Geometry check sheet. Reference: the model listing, model coordinates, mm. A direction names the side the tool comes from. Round coordinates to 2 decimals unless told otherwise and drop trailing zeros. Loops run counter-clockwise (first coordinate to the right, second up) from the corner with the lowest first, then second, coordinate; pieces in that order, holes last. Notation, with made-up numbers: (75, -4) - (119, -4) arc R30 ccw to (119, 22) - close; hole circle Ø5 at (21, 51). An arc over 180 degrees is marked (long way). Write item = value, one per line.
```python
from build123d import *

# Parameters (mm, degrees)
SKETCH1_R           = 49.53
SKETCH1_R_2         = 2.15265
SKETCH1_R_3         = 17.4625
SKETCH1_R_4         = 3.175
BOSS_EXTRUDE1_DEPTH = 3.175
CUT_EXTRUDE1_DEPTH  = 71.117918002


with BuildPart() as part:
    # Sketch1 → Boss-Extrude1 (new body)
    with BuildSketch(Plane(origin=(0, 0, 0), x_dir=(0, 0, -1), z_dir=(1, 0, 0))):
        Circle(SKETCH1_R)
        with Locations((0, 45.085)):
            Circle(SKETCH1_R_2, mode=Mode.SUBTRACT)
        with Locations((31.87990923, 31.87990923)):
            Circle(SKETCH1_R_2, mode=Mode.SUBTRACT)
        with Locations((45.085, 0)):
            Circle(SKETCH1_R_2, mode=Mode.SUBTRACT)
        with Locations((31.87990923, -31.87990923)):
            Circle(SKETCH1_R_2, mode=Mode.SUBTRACT)
        with Locations((0, -45.085)):
            Circle(SKETCH1_R_2, mode=Mode.SUBTRACT)
        with Locations((-31.87990923, -31.87990923)):
            Circle(SKETCH1_R_2, mode=Mode.SUBTRACT)
        with Locations((-45.085, 0)):
            Circle(SKETCH1_R_2, mode=Mode.SUBTRACT)
        with Locations((-31.87990923, 31.87990923)):
            Circle(SKETCH1_R_2, mode=Mode.SUBTRACT)
        Circle(SKETCH1_R_3, mode=Mode.SUBTRACT)
        with Locations((9.720159182, 23.466540126)):
            Circle(SKETCH1_R_4, mode=Mode.SUBTRACT)
        with Locations((23.466540126, -9.720159182)):
            Circle(SKETCH1_R_4, mode=Mode.SUBTRACT)
        with Locations((-9.720159182, -23.466540126)):
            Circle(SKETCH1_R_4, mode=Mode.SUBTRACT)
        with Locations((-23.466540126, 9.720159182)):
            Circle(SKETCH1_R_4, mode=Mode.SUBTRACT)
    extrude(amount=BOSS_EXTRUDE1_DEPTH)

    # Sketch2 → Cut-Extrude1 (cut, through all)
    with BuildSketch(Plane(origin=(3.175, 0, 0), x_dir=(0, 0, -1), z_dir=(1, 0, 0))):
        with BuildLine():
            Line((-20.434868218, -10.637719077), (-33.719928863, -17.553483913))
            ThreePointArc((-33.719928863, -17.553483913), (-34.993654696, -19.123916601), (-34.716893211, -21.126924191))
            ThreePointArc((-34.716893211, -21.126924191), (-13.899698625, -38.189108109), (13.014558026, -38.49975168))
            ThreePointArc((13.014558026, -38.49975168), (14.514078084, -37.143257699), (14.547802162, -35.121501281))
            Line((14.547802162, -35.121501281), (8.816223227, -21.284245682))
            ThreePointArc((8.816223227, -21.284245682), (7.568898247, -19.966485263), (5.760575328, -19.817219233))
            ThreePointArc((5.760575328, -19.817219233), (-7.058440708, -19.392906461), (-17.1511197, -11.478044227))
            ThreePointArc((-17.1511197, -11.478044227), (-18.632321778, -10.430021072), (-20.434868218, -10.637719077))
        make_face()
    extrude(amount=-CUT_EXTRUDE1_DEPTH, mode=Mode.SUBTRACT)


solid = part.part
```
(1) Section check D-D (z = -28). Enter the section's corners in (x, y) (3 decimals), then the cut area to 3 significant figures.
Answers follow:
outline = (0, -40.856) - (3.175, -40.856) - (3.175, 40.856) - (0, 40.856) - close
area = 259 mm²
(2) Scan lines: L1, parallel to Y at x = 0.75, z = 0; L2, parallel to Y at x = 2.65, z = 15.5; L3, parallel to Y at x = 0.8, z = 9.5. Record each from-to range of solid material in increasing order. Write a range as [from, to].
Answers follow:
L1 = [-49.53, -47.24], [-42.93, -40.64], [-20.64, -17.46], [17.46, 42.93], [47.24, 49.53]
L2 = [-47.04, -37.57], [-13.63, -8.04], [8.04, 47.04]
L3 = [-48.61, -39.51], [-18.32, -14.65], [14.65, 48.61]
(3) Section check A-A (z = 0). Enter the section's corners in (x, y) (1 decimal), then the cut area to 3 significant figures.
Answers follow:
outline = (0, -49.5) - (3.2, -49.5) - (3.2, -47.2) - (0, -47.2) - close; (0, -42.9) - (3.2, -42.9) - (3.2, -40.6) - (0, -40.6) - close; (0, -20.6) - (3.2, -20.6) - (3.2, -17.5) - (0, -17.5) - close; (0, 17.5) - (3.2, 17.5) - (3.2, 42.9) - (0, 42.9) - close; (0, 47.2) - (3.2, 47.2) - (3.2, 49.5) - (0, 49.5) - close
area = 113 mm²
(4) Set-up check for faces 1 (the cylindrical face through (1.61, -19.455, 6.887)), 2 (the flat face through (0, 23, 1)): record each of +Z, -Z, +X, -X, +Y, -Y from which the full face is reachable in a straight line by a thin tool's end or side.
Answers follow:
face_1 = +X, -X
face_2 = +Z, -Z, -X, +Y, -Y
(5) Section check B-B (y = 0). Enter the section's corners in (x, z) (1 decimal), then the cut area to 3 significant figures.
Answers follow:
outline = (0, -49.5) - (3.2, -49.5) - (3.2, -47.2) - (0, -47.2) - close; (0, -42.9) - (3.2, -42.9) - (3.2, -17.5) - (0, -17.5) - close; (0, 17.5) - (3.2, 17.5) - (3.2, 42.9) - (0, 42.9) - close; (0, 47.2) - (3.2, 47.2) - (3.2, 49.5) - (0, 49.5) - close
area = 176 mm²
(6) Gauge pin test, flat ends, axial feed: pin 1 (2.5 mm diameter, centred on y = -31.88, z = 31.88, fed in from +X); pin 2 (1 mm diameter, centred on x = 1, y = -17.5, fed in from +Z); pin 3 (1.5 mm diameter, centred on x = 2.5, z = 29, fed in from -Y). Record the tip position at first contact, or that the pin passes through.
Answers follow:
pin_1 = through
pin_2 = 46.52
pin_3 = -40.68
(7) Section check C-C (x = 2.65). State how many separate pieces and enclosed holes the cut face has, then the cut area to 3 significant figures.
Answers follow:
separate_pieces = 1
enclosed_holes = 13
area = 5,630 mm²
(8) Mould release check, pull along Z, two halves, no side actions. Record for faces 3 (the flat face through (3.175, 23, 1)), 4 (the cylindrical face through (1.61, -38.056, 14.26)), 5 (the cylindrical face through (1.57, 14.88, -47.24)): pulls with the +Z half, pulls with the -Z half, needs draft (parallel to the pull), parting line crosses it, or undercut.
Answers follow:
face_3 = needs draft
face_4 = undercut
face_5 = parting line crosses it
